Part print with two shaded views. Sizes in mm from the minimum x, y, z corner. Round coordinates to 2 decimals unless told otherwise and drop trailing zeros. Loops run counter-clockwise (first coordinate to the right, second up) from the corner with the lowest first, then second, coordinate; pieces in that order, holes last. Notation, with made-up numbers: M 46,-32.75 L 73,-32.75 A9 cw 73,-17.75 Z; hole C 12,77 d8. An arc over 180 degrees is marked long. Use a Markdown table: item, result. Add a question column.
Item 1: Wall check: L1, parallel to X at y = 9.5, z = 7.5 (1 decimal); L2, parallel to X at y = 16, z = 1.25 (1 decimal); L3, parallel to Y at x = 10, z = 6.5. Give the ranges that are in metal, low to high. Write a range as from..to.
Item 2: Saw through at C-C on z = 1.5. Write the cut outline in (x, y).
Item 3: Saw through at B-B on y = 29. Write the cut outline in (x, z).
Item 4: Saw through at A-A on x = 30. Write the cut outline in (y, z).
Item 5: Pin check, flat tips, straight feed: P1, Ø4, axis at x = 20, z = 7.5, coming from the +Y side; P2, Ø4, axis at x = 21.5, z = 4, coming from the -Y side. Stop position of each tip, or through.
Item 6: Saw through at D-D on z = 5.5. Write the cut outline in (x, y).
Item 7: Two-plate mould, pull along Y, no slides. Class the marked faces 1, 2 and 3: +Y half, -Y half, draft (parallel to the pull), parting line (faces both ways), or undercut.
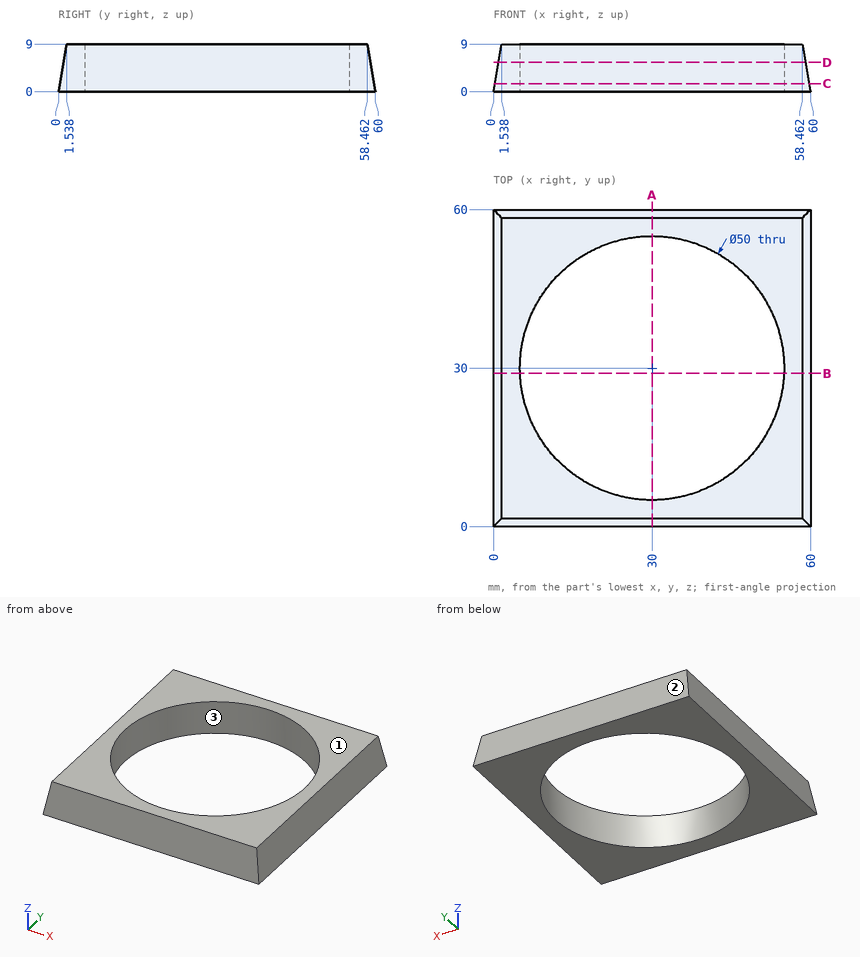
Entries:
| question | item | result |
|---|---|---|
| 1 | L1 | 1.3..15.7, 44.3..58.7 |
| 1 | L2 | 0.2..9.3, 50.7..59.8 |
| 1 | L3 | 1.11..15, 45..58.89 |
| 2 | outline | M 0.26,0.26 L 59.74,0.26 L 59.74,59.74 L 0.26,59.74 Z; hole C 30,30 d50 |
| 3 | outline | M 0,0 L 5.02,0 L 5.02,9 L 1.54,9 Z; M 54.98,0 L 60,0 L 58.46,9 L 54.98,9 Z |
| 4 | outline | M 0,0 L 5,0 L 5,9 L 1.54,9 Z; M 55,0 L 60,0 L 58.46,9 L 55,9 Z |
| 5 | P1 | y = 59.06 |
| 5 | P2 | y = 0.34 |
| 6 | outline | M 0.94,0.94 L 59.06,0.94 L 59.06,59.06 L 0.94,59.06 Z; hole C 30,30 d50 |
| 7 | face 1 | draft |
| 7 | face 2 | +Y half |
| 7 | face 3 | undercut |
